```python
from build123d import *

# Parameters (mm, degrees)
BOSS_EXTRUDE1_DEPTH  = 35
M4_CLEARANCE_HOLE1_D = 4.5
M4_CLEARANCE_HOLE2_D = 4.8


with BuildPart() as part:
    # Sketch1 → Boss-Extrude1 (new body)
    with BuildSketch(Plane.XY):
        Polygon((0, 0), (12.7, 0), (12.7, -1.524), (1.524, -1.524), (1.524, -12.7), (0, -12.7), align=None)
    extrude(amount=BOSS_EXTRUDE1_DEPTH)

    # M4 Clearance Hole1 (through all)
    with Locations(Plane(origin=(0, 0, 0), x_dir=(1, 0, 0), z_dir=(0, 1, 0))):
        with Locations((9, -5)):
            Hole(M4_CLEARANCE_HOLE1_D / 2)

    # M4 Clearance Hole2 (through all)
    with Locations(Plane.ZY):
        with Locations((15, -6.35), (28.5, -6.35)):
            Hole(M4_CLEARANCE_HOLE2_D / 2)


solid = part.part
```
The listing builds one solid part. Answer for the finished solid, in the listing's coordinates (mm). A direction names the side the tool comes from. Give positions to 0.01 mm unless a question says otherwise; leave off trailing zeros. Loops run counter-clockwise (first coordinate to the right, second up) from the corner with the lowest first, then second, coordinate; pieces in that order, holes last. Notation, with made-up numbers: (43, 37) - (61, 37) arc R30 cw to (61, 63) - close; hole circle Ø11 at (1.5, -27). An arc over 180 degrees is marked (long way). Answer as CSV lines item,"result". Start each with the question number.
Item 1: The mould has two halves that part along Z. Classify faces 1 (the face through (4, -1, 0)), 2 (the face through (0.773, -6.244, 17.398)), 3 (the face through (0.773, -7.269, 26.283)), 4 (the face through (12.7, -1, 17)): +Z half, -Z half, draft (parallel to the pull), parting line (faces both ways), or undercut.
Item 2: A cutting plane is placed at A-A on y = -6.35. Determine the outline of the cut face in (x, z).
Item 3: A cutting plane is placed at D-D on z = 5. Determine the outline of the cut face in (x, y).
Item 4: A cutting plane is placed at B-B on z = 28.5. Determine the outline of the cut face in (x, y).
Item 5: Find the intervals of material crossed by line 1 (Y direction, x = 0.75, z = 28.5); line 2 (Z direction, x = 9, y = -0.7); line 3 (X direction, y = -4.75, z = 9.5), in increasing order. Write a range as from..to.
Item 6: Each of these flat-tipped pins is pushed along its axis until it touches: pin 1 (3.5 mm diameter, centred on y = -6, z = 22, fed in from +X); pin 2 (7 mm diameter, centred on x = 9, z = 5, fed in from +Y); pin 3 (3 mm diameter, centred on y = -6.35, z = 15, fed in from +X); pin 4 (2 mm diameter, centred on x = 6.5, z = 11.5, fed in from -Y). Where does it stop, or does it pass through?
Item 7: For faces 5 (the face through (7, -1.524, 17)), 6 (the face through (1, -12.7, 17)), determine the directions among +Z, -Z, +X, -X, +Y, -Y from which every point of the face is accessible in a straight line to the end or side of a thin tool.
Item 8: A cutting plane is placed at C-C on x = 9.25. Determine the outline of the cut face in (y, z), then the cut area to 3 significant figures.
Found:
1,face 1,"-Z half"
1,face 2,"undercut"
1,face 3,"undercut"
1,face 4,"draft"
2,outline,"(0, 0) - (1.52, 0) - (1.52, 12.6) - (0, 12.6) - close; (0, 17.4) - (1.52, 17.4) - (1.52, 26.1) - (0, 26.1) - close; (0, 30.9) - (1.52, 30.9) - (1.52, 35) - (0, 35) - close"
3,outline,"(0, -12.7) - (1.52, -12.7) - (1.52, -1.52) - (6.75, -1.52) - (6.75, 0) - (0, 0) - close; (11.25, -1.52) - (12.7, -1.52) - (12.7, 0) - (11.25, 0) - close"
4,outline,"(0, -12.7) - (1.52, -12.7) - (1.52, -8.75) - (0, -8.75) - close; (0, -3.95) - (1.52, -3.95) - (1.52, -1.52) - (12.7, -1.52) - (12.7, 0) - (0, 0) - close"
5,line 1,"y = -12.7..-8.75, -3.95..0"
5,line 2,"z = 0..2.75, 7.25..35"
5,line 3,"x = 0..1.52"
6,pin 1,"stops at x = 1.52"
6,pin 2,"stops at y = 0"
6,pin 3,"passes through"
6,pin 4,"stops at y = -1.52"
7,face 5,"+Z, -Z, +X, -Y"
7,face 6,"+Z, -Z, +X, -X, -Y"
8,outline,"(-1.52, 0) - (0, 0) - (0, 2.76) - (-1.52, 2.76) - close; (-1.52, 7.24) - (0, 7.24) - (0, 35) - (-1.52, 35) - close"
8,area,"46.5 mm^2"
